Here's how the part is built. I have some questions about the finished solid (model axes, mm). Round coordinates to 2 decimals unless told otherwise and drop trailing zeros. Order: outer loops, then holes, each group sorted by start corner. A loop starts at its lowest first (then second) coordinate and runs counter-clockwise, first axis right, second up.
```python
from build123d import *

# Parameters (mm, degrees)
F0_W     = 239
F0_H     = 43
F1_DEPTH = 2
F2_W     = 237
F2_H     = 41
F3_DEPTH = 2
F4_W     = 239
F4_H     = 43
F5_DEPTH = 2
F6_W     = 247
F6_H     = 50
F7_DEPTH = 3


with BuildPart() as f1:
    # F0 (on Top) → F1 (new body)
    with BuildSketch(Plane.XY):
        Rectangle(F0_W, F0_H)
    extrude(amount=F1_DEPTH)

    # F2 (on face) → F3 (join)
    with BuildSketch(Plane.XY.offset(2)):
        Rectangle(F2_W, F2_H)
    extrude(amount=F3_DEPTH)

    # F4 (on face) → F5 (join)
    with BuildSketch(Plane.XY.offset(4)):
        Rectangle(F4_W, F4_H)
    extrude(amount=F5_DEPTH)

    # F6 (on face) → F7 (join)
    with BuildSketch(Plane.XY.offset(6)):
        Rectangle(F6_W, F6_H)
    extrude(amount=F7_DEPTH)


solid = f1.part
```
1) If we section it at B-B (x = -83): Write out the boundary of the cut face in (y, z), plus the area to 3 significant figures.
2) I'm going to push flat-ended pins straight in: pin 1 (6 mm diameter, centred on x = -10.5, y = 20, fed in from -Z); pin 2 (1 mm diameter, centred on y = 7.5, z = 5, fed in from +X); pin 3 (1.6 mm diameter, centred on y = -3, z = 1, fed in from -X); pin 4 (2 mm diameter, centred on x = -51, z = 3.5, fed in from -Y). Where does each tip first touch, or does it pass through?
3) If we section it at A-A (y = -11): Write out the boundary of the cut face in (x, z).
4) I need wall thicknesses on line 1 (Z direction, x = -28.5, y = 23); line 2 (Y direction, x = -48, z = 0.5); line 3 (X direction, y = 18, z = 3.5). Which ranges of each line are inside material? Lowest first, please.
Solutions:
1. outline: (-25, 6) - (-21.5, 6) - (-21.5, 4) - (-20.5, 4) - (-20.5, 2) - (-21.5, 2) - (-21.5, 0) - (21.5, 0) - (21.5, 2) - (20.5, 2) - (20.5, 4) - (21.5, 4) - (21.5, 6) - (25, 6) - (25, 9) - (-25, 9) - close
1. area: 404 mm2
2. pin 1: stops at z = 0
2. pin 2: stops at x = 119.5
2. pin 3: stops at x = -119.5
2. pin 4: stops at y = -21.5
3. outline: (-123.5, 6) - (-119.5, 6) - (-119.5, 4) - (-118.5, 4) - (-118.5, 2) - (-119.5, 2) - (-119.5, 0) - (119.5, 0) - (119.5, 2) - (118.5, 2) - (118.5, 4) - (119.5, 4) - (119.5, 6) - (123.5, 6) - (123.5, 9) - (-123.5, 9) - close
4. line 1: z = 6 to 9
4. line 2: y = -21.5 to 21.5
4. line 3: x = -118.5 to 118.5
